Could you check a few things on this model? Use its own coordinates, in mm. Face numbers are marked on the shaded views. A direction names the side the tool comes from. Round coordinates to 2 decimals unless told otherwise and drop trailing zeros. Order: outer loops, then holes, each group sorted by start corner. A loop starts at its lowest first (then second) coordinate and runs counter-clockwise, first axis right, second up. Notation, with made-up numbers: M 87.5,6 L 143.5,6 A19 ccw 143.5,11 Z; hole C 10.25,86.5 d3. An arc over 180 degrees is marked long. Write each question's results on one line, items separated by ' | '. Start each with the question number.
1. Please list where these lines run through material, in increasing order: L1, parallel to Y at x = 5.5, z = 4; L2, parallel to Y at x = -1, z = -6; L3, parallel to Z at x = 5, y = 25.5 (3 decimals).
2. I'm going to push flat-ended pins straight in: pin 1 (1.9 mm diameter, centred on x = 0.5, z = 8.5, fed in from -Y); pin 2 (1 mm diameter, centred on y = 20, z = 6.5, fed in from +X); pin 3 (1.2 mm diameter, centred on y = 25.5, z = 9, fed in from -X). Where does each tip first touch, or does it pass through?
3. We'd pull the mould along Y, two halves only. Please class the marked faces 4, 5, 6 and 7: released by +Y, released by -Y, zero draft, split by the parting line, or undercut.
4. Suppose I cut it at A-A on z = -6.25. Write out the boundary of the cut face in (x, y), and give its area (3 significant figures).
5. For the marked faces 1, 2 and 3, which set-ups out of +Z, -Z, +X, -X, +Y, -Y let a thin tool reach every point of the face, with its end or its side?
6. Suppose I cut it at C-C on y = 25.5. Write out the boundary of the cut face in (x, z).
7. Suppose I cut it at D-D on z = 2. Write out the boundary of the cut face in (x, y).
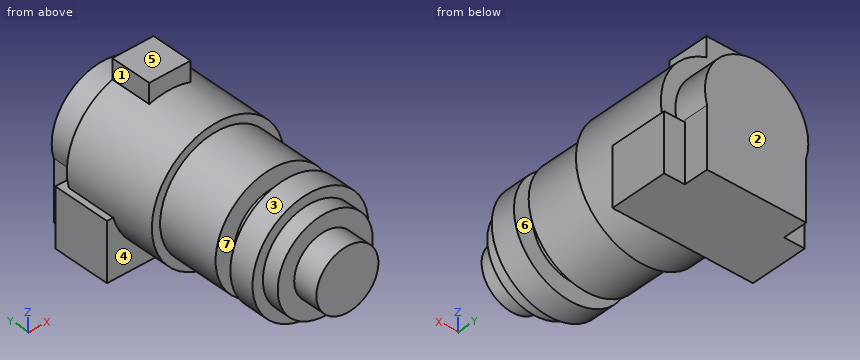
Autodesk Inventor part; units mm, degrees
ref_plane "YZ Plane" through (0, 0, 0) normal (1, 0, 0) x (0, 1, 0)
ref_plane "XZ Plane" through (0, 0, 0) normal (0, 1, 0) x (-1, 0, 0)
ref_plane "XY Plane" through (0, 0, 0) normal (0, 0, 1) x (1, 0, 0)
sketch "Sketch1" plane through (0, 0, 0) normal (0, 1, 0) x (-1, 0, 0)
  circle A0 centre (0, 0) radius 3.75
  dimension "d0" = 7.5
extrude "Extrusion1" add sketch "Sketch1" along normal blind 5
sketch "Sketch2" plane through (0, 5, 0) normal (0, 1, 0) x (1, 0, 0)
  circle A0 centre (0, 0) radius 7
  dimension "d3" = 14
extrude "Extrusion2" add sketch "Sketch2" along normal blind 4
sketch "Sketch3" plane through (0, 9, 0) normal (0, 1, 0) x (1, 0, 0)
  circle A0 centre (0, 0) radius 4.75
  dimension "d6" = 9.5
extrude "Extrusion3" add sketch "Sketch3" along normal blind 4
sketch "Sketch4" plane through (0, 0, 0) normal (1, 0, 0) x (0, 1, 0)
  line L0 (5, -7) -> (5, 7)
  line L1 (9, -7) -> (9, 7)
  line L2 (13, -4.75) -> (13, 4.75)
  line L3 (0, -3.75) -> (0, 3.75)
  point P0 (0, 0)
  dimension "d9" = 4
  dimension "d10" = 4
  dimension "d11" = 5
sketch "Sketch5" plane through (0, 13, 0) normal (0, 1, 0) x (1, 0, 0)
  circle A0 centre (0, 0) radius 7
  dimension "d12" = 14
extrude "Extrusion4" add sketch "Sketch5" along normal blind 4.5
sketch "Sketch6" plane through (0, 17.5, 0) normal (0, 1, 0) x (1, 0, 0)
  circle A0 centre (0, 0) radius 8
  dimension "d15" = 16
extrude "Extrusion5" add sketch "Sketch6" along normal blind 11.5
sketch "Sketch7" plane through (0, 29, 0) normal (0, 1, 0) x (1, 0, 0)
  circle A0 centre (0, 0) radius 6.25
  dimension "d18" = 12.5
extrude "Extrusion6" add sketch "Sketch7" along normal blind 25
sketch "Sketch8" plane through (0, 0, 0) normal (1, 0, 0) x (0, 1, 0)
  line L0 (54, -6.25) -> (54, 6.25)
  line L1 (0, -3.75) -> (0, 3.75)
  line L2 (29, -8) -> (29, 8)
  line L3 (17.5, -8) -> (17.5, 8)
  point P0 (0, 0)
  point P1 (0, 0)
  dimension "d21" = 54
  dimension "d22" = 29
  dimension "d23" = 17.5
sketch "Sketch9" plane through (0, 54, 0) normal (0, 1, 0) x (1, 0, 0)
  circle A0 centre (0, 0) radius 7
  dimension "d24" = 14
extrude "Extrusion7" add sketch "Sketch9" along normal blind 10
sketch "Sketch10" plane through (0, 0, 0) normal (1, 0, 0) x (0, 1, 0)
  line L0 (64, -7) -> (64, 7)
  line L1 (0, -3.75) -> (0, 3.75)
  point P0 (0, 0)
  dimension "d27" = 64
sketch "Sketch11" plane through (0, 64, 0) normal (0, 1, 0) x (1, 0, 0)
  circle A0 centre (0, 0) radius 7
  dimension "d28" = 14
extrude "Extrusion8" add sketch "Sketch11" along normal blind 9
sketch "Sketch12" plane through (0, 73, 0) normal (0, 1, 0) x (1, 0, 0)
  circle A0 centre (0, 0) radius 4.5
  dimension "d31" = 9
extrude "Extrusion9" add sketch "Sketch12" along normal blind 1
sketch "Sketch13" plane through (0, 0, 0) normal (1, 0, 0) x (0, 1, 0)
  point P0 (0, 0)
sketch "Sketch14" plane through (0, 0, 0) normal (1, 0, 0) x (0, 1, 0)
  line L0 (73, -7) -> (73, 7)
  line L1 (0, -3.75) -> (0, 3.75)
  line L2 (74, -4.5) -> (74, 4.5)
  point P0 (0, 0)
  point P1 (0, 0)
  dimension "d34" = 73
  dimension "d35" = 74
sketch "Sketch15" plane through (0, 74, 0) normal (0, 1, 0) x (1, 0, 0)
  circle A0 centre (0, 0) radius 7
  dimension "d36" = 14
extrude "Extrusion10" add sketch "Sketch15" along normal blind 11.5
sketch "Sketch16" plane through (0, 0, 0) normal (1, 0, 0) x (0, 1, 0)
  line L0 (85.5, -7) -> (85.5, 7)
  line L1 (0, -3.75) -> (0, 3.75)
  point P0 (0, 0)
  dimension "d39" = 85.5
sketch "Sketch17" plane through (0, 0, 0) normal (1, 0, 0) x (0, 1, 0)
  line L0 (23, -9) -> (30, -9)
  line L1 (0, -3.75) -> (0, 3.75)
  line L2 (23, -9) -> (23, -2)
  line L3 (54, 7) -> (73, 7)
  line L4 (23, -2) -> (30, -2)
  line L5 (30, -2) -> (30, -9)
  point P0 (0, 0)
  point P1 (0, 0)
  point P2 (26.5, -9)
  dimension "d40" = 7
  dimension "d41" = 23
  dimension "d42" = 7
  dimension "d43" = 9
extrude "Extrusion11" add sketch "Sketch17" along normal mid plane 17
sketch "Sketch18" plane through (0, 0, 0) normal (1, 0, 0) x (0, 1, 0)
  line L0 (24, 10) -> (29, 10)
  line L1 (29, 10) -> (29, 6)
  line L2 (29, 6) -> (24, 6)
  line L3 (17.5, 8) -> (29, 8)
  line L4 (24, 6) -> (24, 10)
  line L5 (0, -3.75) -> (0, 3.75)
  point P0 (0, 0)
  point P1 (24, 8)
  point P2 (0, 0)
  point P3 (26.5, 10)
  dimension "d46" = 5
  dimension "d47" = 4
  dimension "d48" = 24
  dimension "d49" = 10
extrude "Extrusion12" add sketch "Sketch18" along normal mid plane 5
sketch "Sketch19" plane through (8.5, 0, 0) normal (1, 0, 0) x (0, 0, -1)
  line L0 (3.75, 0) -> (-3.75, 0)
  point P0 (0, 0)
  point P1 (9, 23)
  dimension "d52" = 23
sketch "Sketch20" plane through (8.5, 30, -9) normal (0, 0, -1) x (-1, 0, 0)
  line L0 (14.4214, 0) -> (2.5786, 0)
  line L1 (8.5, 0) -> (2.5, 0)
  line L2 (2.5, 0) -> (2.5, 29)
  line L3 (1.5, 24) -> (1.5, 43)
  line L4 (2.5, 29) -> (14.5, 29)
  line L5 (14.5, 29) -> (14.5, 0)
  line L6 (14.5, 0) -> (2.5, 0)
  point P0 (8.5, -30)
  point P1 (2.5786, 0)
  dimension "d53" = 6
  dimension "d54" = 29
  dimension "d55" = 90
  dimension "d56" = 12
  dimension "d57" = 29
  dimension "d58" = 90
extrude "Extrusion13" add sketch "Sketch20" against normal blind 9
sketch "Sketch21" plane through (8.5, 23, -9) normal (0, 0, -1) x (-1, 0, 0)
  point P0 (8.5, -23)
sketch "Sketch22" plane through (0, 13, 0) normal (0, -1, 0) x (1, 0, 0)
  circle A0 centre (0, 0) radius 7
extrude "Extrusion14" add sketch "Sketch22" along normal blind 3
sketch "Sketch23" plane through (0, 9, 0) normal (0, 1, 0) x (1, 0, 0)
  circle A0 centre (0, 0) radius 3.75
  circle A1 centre (0, 0) radius 7
  circle A2 centre (0, 0) radius 7
  circle A3 centre (0, 0) radius 4.75
  dimension "d63" = 14
  dimension "d64" = 9.5
extrude "Extrusion15" cut sketch "Sketch23" against normal blind 1 contours A1
sketch "Sketch24" plane through (0, 5, 0) normal (0, -1, 0) x (1, 0, 0)
  circle A0 centre (0, 0) radius 5.75
  dimension "d67" = 11.5
extrude "Extrusion16" add sketch "Sketch24" along normal blind 2
sketch "Sketch25" plane through (0, 85.5, 0) normal (0, 1, 0) x (1, 0, 0)
  circle A0 centre (0, 0) radius 7
extrude "Extrusion17" cut sketch "Sketch25" against normal blind 6.5
sketch "Sketch26" plane through (0, 0, 0) normal (1, 0, 0) x (0, 1, 0)
  line L0 (79, 7) -> (79, -7)
  line L1 (0, -3.75) -> (0, 3.75)
  point P0 (0, 0)
  dimension "d72" = 79
sketch "Sketch27" plane through (0, 79, 0) normal (0, 1, 0) x (1, 0, 0)
  point P0 (0, 0)
sketch "Sketch28" plane through (0, 79, 0) normal (0, 1, 0) x (1, 0, 0)
  circle A0 centre (0, 0) radius 17.2984
extrude "Extrusion18" cut sketch "Sketch28" against normal blind 13
extrude "Extrusion19" cut sketch "Sketch28" against normal blind 46
equation "\"BendRadius\" = Thickness"
equation "\"BendReliefWidth\" = Thickness"
equation "\"BendReliefDepth\" = 0.5 * Thickness"
equation "\"CornerReliefSize\" = 4 * Thickness"
equation "\"MinimumRemnant\" = 2 * Thickness"
equation "\"TransitionRadius\" = BendRadius"
equation "\"JacobiRadiusSize\" = BendRadius"
equation "\"GapSize\" = Thickness"
properties part number "injector carcasa - 3"
Filled sheet:
1) L1: y = 5 to 8, 10 to 29 | L2: y = 5 to 8, 10 to 33 | L3: z = -9 to 6.245
2) pin 1: stops at y = 17.5 | pin 2: stops at x = 5.29 | pin 3: stops at x = -2.5
3) face 4: released by -Y | face 5: zero draft | face 6: undercut | face 7: undercut
4) outline: M -8.5,23 L -4.99,23 L -4.99,17.5 L -3.15,17.5 L -3.15,10 L 3.15,10 L 3.15,17.5 L 4.99,17.5 L 4.99,23 L 8.5,23 L 8.5,30 L 6,30 L 6,33 L -6,33 L -6,30 L -8.5,30 Z; M -3.15,5 L 3.15,5 L 3.15,8 L -3.15,8 Z | area: 276 mm^2
5) face 1: +Z, -X, +Y, -Y | face 2: +Z, -Z, +X, -X, +Y | face 3: -Y
6) outline: M -8.5,-9 L 8.5,-9 L 8.5,-2 L 7.75,-2 A8 ccw 2.5,7.6 L 2.5,10 L -2.5,10 L -2.5,7.6 A8 ccw -7.75,-2 L -8.5,-2 Z
7) outline: M -7.75,17.5 L -6.71,17.5 L -6.71,10 L -4.31,10 L -4.31,8 L -6.71,8 L -6.71,5 L -5.39,5 L -5.39,3 L -3.17,3 L -3.17,0 L 3.17,0 L 3.17,3 L 5.39,3 L 5.39,5 L 6.71,5 L 6.71,8 L 4.31,8 L 4.31,10 L 6.71,10 L 6.71,17.5 L 7.75,17.5 L 7.75,29 L 5.92,29 L 5.92,33 L -5.92,33 L -5.92,29 L -7.75,29 Z
